Study the drawing (mm; zero at the part's minimum x, y, z) and answer. Give positions to 0.01 mm unless a question says otherwise; leave off trailing zeros. Write each loop counter-clockwise with the first axis right and the second up, starting at its lowest first coordinate (ties: lowest second). Pieces come first, ordered by that corner, then holes. Notation, with made-up numbers: M 38,81.5 L 95,81.5 A20 cw 95,118.5 Z; hole C 38.25,65 d8. An arc over 180 degrees is marked long. Use a Markdown table: item, result. Add a question column.
Item 1: A cutting plane is placed at C-C on x = 17. Determine the outline of the cut face in (y, z), then the cut area to 3 significant figures.
Item 2: Consider probe 1 along Z at (x, y) = (16.25, 11); probe 2 along Z at (x, y) = (17.25, 13.5). Determine where each line is inside the solid, lowest interval first. Write a range as [from, to].
Item 3: The mould has two halves that part along Z. Classify the marked faces 1, 2 and 3: pulls with the +Z half, pulls with the -Z half, needs draft (parallel to the pull), parting line crosses it, or undercut.
Item 4: Given P1, Ø3, axis at x = 17.5, z = 3.5, coming from the +Y side; P2, Ø12, axis at x = 14, y = 7.5, coming from the +Z side; P3, Ø1.5, axis at x = 12, z = 15.5, coming from the +Y side, each flat-ended and moving along its own axis, determine where each tip first touches the part or whether it passes through.
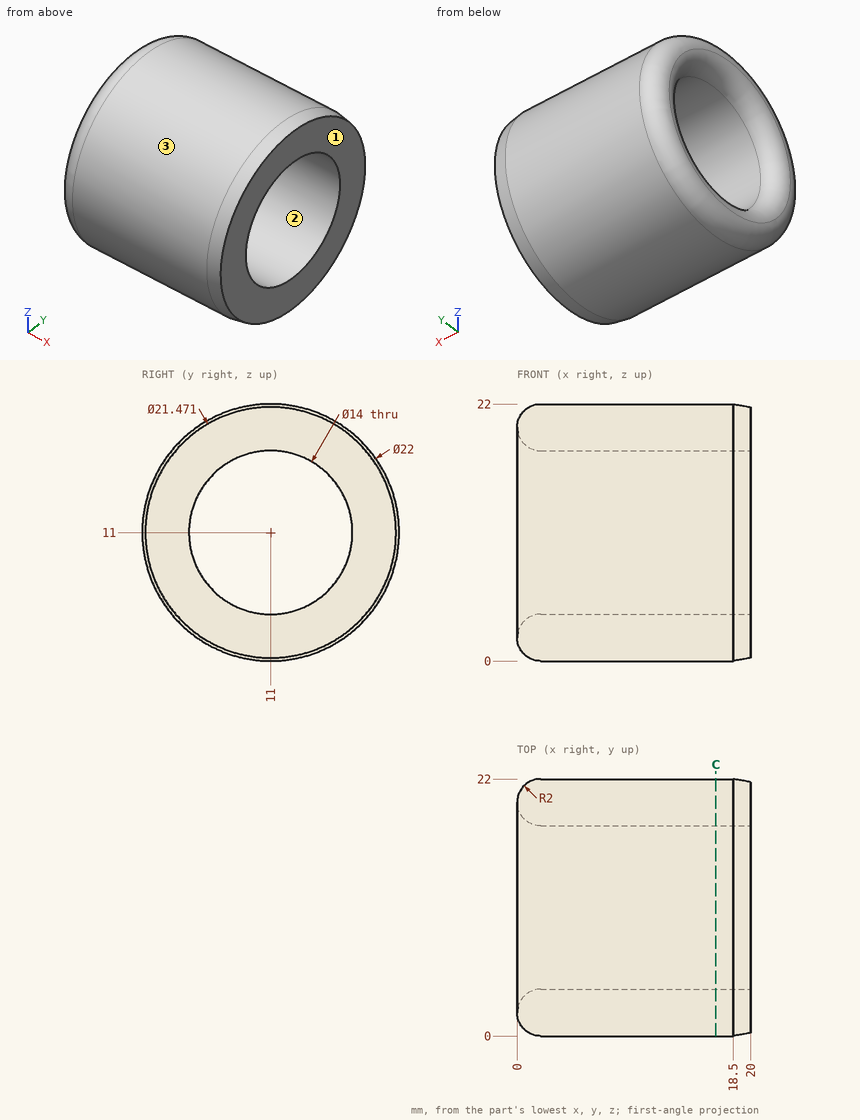
Filled in:
| question | item | result |
|---|---|---|
| 1 | outline | C 11,11 d22; hole C 11,11 d14 |
| 1 | area | 226 mm² |
| 2 | probe 1 | [0, 4], [18, 22] |
| 2 | probe 2 | [0.29, 4.46], [17.54, 21.71] |
| 3 | face 1 | needs draft |
| 3 | face 2 | undercut |
| 3 | face 3 | parting line crosses it |
| 4 | P1 | y = 20.22 |
| 4 | P2 | z = 22 |
| 4 | P3 | y = 21.34 |
